```python
from build123d import *

# Parameters (mm, degrees)
F0_W     = 25
F0_H     = 280
F0_H_2   = 25
F1_DEPTH = 1


with BuildPart() as f1:
    # F0 (on Top) → F1 (new body)
    with BuildSketch(Plane.XY):
        with Locations((12.591098, 165.051688)):
            Rectangle(F0_W, F0_H)
        with Locations((37.591098, 165.051688)):
            Rectangle(F0_W, F0_H)
        with Locations((62.591098, 165.051688)):
            Rectangle(F0_W, F0_H)
        with BuildLine():
            Line((75.091098, 25.051688), (50.091098, 25.051688))
            Line((50.091098, 25.051688), (50.091098, 0.051688))
            ThreePointArc((50.091098, 0.051688), (67.768768, 7.374019), (75.091098, 25.051688))
        make_face()
        with Locations((37.591098, 12.551688)):
            Rectangle(F0_W, F0_H_2)
        with BuildLine():
            Line((25.091098, 0.051688), (25.091098, 25.051688))
            Line((25.091098, 25.051688), (0.091098, 25.051688))
            ThreePointArc((0.091098, 25.051688), (7.413429, 7.374019), (25.091098, 0.051688))
        make_face()
        with BuildLine():
            Line((0.091098, 305.051688), (25.091098, 305.051688))
            Line((25.091098, 305.051688), (25.091098, 330.051688))
            ThreePointArc((25.091098, 330.051688), (7.413429, 322.729358), (0.091098, 305.051688))
        make_face()
        with Locations((37.591098, 317.551688)):
            Rectangle(F0_W, F0_H_2)
        with BuildLine():
            Line((50.091098, 330.051688), (50.091098, 305.051688))
            Line((50.091098, 305.051688), (75.091098, 305.051688))
            ThreePointArc((75.091098, 305.051688), (67.768768, 322.729358), (50.091098, 330.051688))
        make_face()
    extrude(amount=F1_DEPTH)


solid = f1.part
```
The listing builds one solid part. Answer for the finished solid, in the listing's coordinates (mm). Round coordinates to 2 decimals unless told otherwise and drop trailing zeros. Write each loop counter-clockwise with the first axis right and the second up, starting at its lowest first coordinate (ties: lowest second). Pieces come first, ordered by that corner, then holes. Notation, with made-up numbers: (-33.75, 42.5) -> (3.25, 42.5) arc R28 ccw to (3.25, 78.5) -> close; hole circle Ø3 at (54, -11). An arc over 180 degrees is marked (long way). Answer as a JSON object with one key per item and string values. Group by question number.
Q1. Section A-A (z = 0.6) is taken. Write down the section's boundary in (x, y), plus the area to 3 significant figures.
Q2. Section B-B (x = 66) is taken. Write down the section's boundary in (y, z).
Q3. Section C-C (x = 12) is taken. Write down the section's boundary in (y, z).
Q4. Straight lines are drawn through the part: line 1 along Y through (x, z) = (51, 0.4); line 2 along Y through (x, z) = (61.5, 0.8); line 3 along X through (y, z) = (317.5, 0.95). For each, find the intervals that lie inside material, in ascending order.
Check values:
{
 "1": {"outline": "(0.09, 25.05) arc R25 ccw to (25.09, 0.05) -> (50.09, 0.05) arc R25 ccw to (75.09, 25.05) -> (75.09, 305.05) arc R25 ccw to (50.09, 330.05) -> (25.09, 330.05) arc R25 ccw to (0.09, 305.05) -> close", "area": "24,200 mm^2"},
 "2": {"outline": "(5.77, 0) -> (324.34, 0) -> (324.34, 1) -> (5.77, 1) -> close"},
 "3": {"outline": "(3.75, 0) -> (326.35, 0) -> (326.35, 1) -> (3.75, 1) -> close"},
 "4": {"line 1": "0.07 to 330.04", "line 2": "2.81 to 327.3", "line 3": "3.41 to 71.77"}
}
